Design review of the part built by this model. Coordinates are the model's own, in mm. Give positions to 0.01 mm unless a question says otherwise; leave off trailing zeros. Loops run counter-clockwise (first coordinate to the right, second up) from the corner with the lowest first, then second, coordinate; pieces in that order, holes last.
Autodesk Inventor part; units mm, degrees
ref_plane "YZ Plane" through (0, 0, 0) normal (1, 0, 0) x (0, 1, 0)
ref_plane "XZ Plane" through (0, 0, 0) normal (0, 1, 0) x (-1, 0, 0)
ref_plane "XY Plane" through (0, 0, 0) normal (0, 0, 1) x (1, 0, 0)
sketch "Sketch1" plane through (0, 0, 0) normal (0, 0, 1) x (1, 0, 0)
  line L0 (6, 225.5) -> (202, 225.5)
  line L1 (242, 185.5) -> (242, -10.5)
  line L2 (202, -50.5) -> (6, -50.5)
  line L3 (-34, -10.5) -> (-34, 185.5)
  line L4 (208, 237.5) -> (0, 237.5) construction
  line L5 (-46, 191.5) -> (-46, -16.5) construction
  arc A0 (0, 237.5) -> (-46, 191.5) centre (0, 191.5) ccw construction
  arc A1 (6, 225.5) -> (-34, 185.5) centre (6, 185.5) ccw
  arc A2 (242, 185.5) -> (202, 225.5) centre (202, 185.5) ccw
  arc A3 (202, -50.5) -> (242, -10.5) centre (202, -10.5) ccw
  arc A4 (-34, -10.5) -> (6, -50.5) centre (6, -10.5) ccw
  line L6 (51.5, 191.5) -> (16.5, 191.5)
  line L7 (16.5, 191.5) -> (16.5, 187.5)
  line L8 (51.5, 187.5) -> (16.5, 187.5)
  line L9 (51.5, 191.5) -> (51.5, 187.5)
  line L10 (121.5, 191.5) -> (86.5, 191.5)
  line L11 (86.5, 191.5) -> (86.5, 187.5)
  line L12 (121.5, 187.5) -> (86.5, 187.5)
  line L13 (121.5, 191.5) -> (121.5, 187.5)
  line L14 (191.5, 191.5) -> (156.5, 191.5)
  line L15 (156.5, 191.5) -> (156.5, 187.5)
  line L16 (191.5, 187.5) -> (156.5, 187.5)
  line L17 (191.5, 191.5) -> (191.5, 187.5)
  line L18 (208, 140) -> (208, 175)
  line L19 (208, 175) -> (204, 175)
  line L20 (204, 140) -> (204, 175)
  line L21 (208, 140) -> (204, 140)
  line L22 (208, 70) -> (208, 105)
  line L23 (208, 105) -> (204, 105)
  line L24 (204, 70) -> (204, 105)
  line L25 (208, 70) -> (204, 70)
  line L26 (208, 0) -> (208, 35)
  line L27 (208, 35) -> (204, 35)
  line L28 (204, 0) -> (204, 35)
  line L29 (208, 0) -> (204, 0)
  line L30 (156.5, -16.5) -> (191.5, -16.5)
  line L31 (191.5, -16.5) -> (191.5, -12.5)
  line L32 (156.5, -12.5) -> (191.5, -12.5)
  line L33 (156.5, -16.5) -> (156.5, -12.5)
  line L34 (86.5, -16.5) -> (121.5, -16.5)
  line L35 (121.5, -16.5) -> (121.5, -12.5)
  line L36 (86.5, -12.5) -> (121.5, -12.5)
  line L37 (86.5, -16.5) -> (86.5, -12.5)
  line L38 (16.5, -16.5) -> (51.5, -16.5)
  line L39 (51.5, -16.5) -> (51.5, -12.5)
  line L40 (16.5, -12.5) -> (51.5, -12.5)
  line L41 (16.5, -16.5) -> (16.5, -12.5)
  line L42 (0, 35) -> (0, 0)
  line L43 (0, 0) -> (4, 0)
  line L44 (4, 35) -> (4, 0)
  line L45 (0, 35) -> (4, 35)
  line L46 (0, 105) -> (0, 70)
  line L47 (0, 70) -> (4, 70)
  line L48 (4, 105) -> (4, 70)
  line L49 (0, 105) -> (4, 105)
  line L50 (0, 175) -> (0, 140)
  line L51 (0, 140) -> (4, 140)
  line L52 (4, 175) -> (4, 140)
  line L53 (0, 175) -> (4, 175)
  circle A5 centre (43, 152.5) radius 7.5
  line L54 (4, 180) -> (4, 165)
  line L55 (24, 7.5) -> (28, 7.5)
  line L56 (28, 7.5) -> (28, 47.5)
  line L57 (28, 47.5) -> (24, 47.5)
  line L58 (24, 47.5) -> (24, 7.5)
  line L59 (180, 7.5) -> (184, 7.5)
  line L60 (184, 7.5) -> (184, 47.5)
  line L61 (184, 47.5) -> (180, 47.5)
  line L62 (180, 47.5) -> (180, 7.5)
  line L63 (180, 127.5) -> (184, 127.5)
  line L64 (184, 127.5) -> (184, 167.5)
  line L65 (184, 167.5) -> (180, 167.5)
  line L66 (180, 167.5) -> (180, 127.5)
  line L67 (24, 127.5) -> (28, 127.5)
  line L68 (28, 127.5) -> (28, 167.5)
  line L69 (28, 167.5) -> (24, 167.5)
  line L70 (24, 167.5) -> (24, 127.5)
  line L71 (104, 187.5) -> (104, -12.5) construction
  circle A6 centre (26, 107.5) radius 1.5
  circle A7 centre (26, 67.5) radius 1.5
  circle A8 centre (182, 107.5) radius 1.5
  circle A9 centre (182, 67.5) radius 1.5
  line L72 (26, 127.5) -> (26, 107.5) construction
  line L73 (26, 67.5) -> (26, 47.5) construction
  line L74 (26, 107.5) -> (26, 87.5) construction
  line L75 (26, 87.5) -> (26, 67.5) construction
  line L76 (51.5, 191.5) -> (86.5, 187.5) construction
  line L77 (121.5, 187.5) -> (156.5, 191.5) construction
  circle A10 centre (69, 189.5) radius 1.5
  circle A11 centre (139, 189.5) radius 1.5
  circle A12 centre (2, 122.5) radius 1.5
  circle A13 centre (2, 52.5) radius 1.5
  circle A14 centre (69, -14.5) radius 1.5
  circle A15 centre (139, -14.5) radius 1.5
  circle A16 centre (206, 52.5) radius 1.5
  circle A17 centre (206, 122.5) radius 1.5
  point P0 (104, 237.5)
  point P1 (104, 225.5)
  point P2 (-34, 87.5)
  point P3 (-46, 87.5)
  point P4 (-24, 191.5)
  point P5 (4, 172.5)
  point P6 (182, 127.5)
  point P7 (182, 47.5)
  point P8 (104, 87.5)
  dimension "d0" = 10
  dimension "d2" = 40
  dimension "d4" = 15
  dimension "d6" = 4
  dimension "d7" = 40
  dimension "d9" = 20
  dimension "d10" = 4
  dimension "d11" = 40
  dimension "d12" = 4
  dimension "d13" = 40
  dimension "d14" = 4
  dimension "d15" = 40
  dimension "d16" = 20
  dimension "d17" = 15
  dimension "d18" = 15
  dimension "d19" = 20
  dimension "d22" = 3
  dimension "d24" = 3
  dimension "d27" = 360
extrude "Extrusion1" add sketch "Sketch1" along normal blind 4
properties part number "Cover" material "MDF Medium Density Fiberboard"
Q1. Take a section at C-C (z = 0.8). Give the number of separate pieces and of enclosed holes in the cut face, plus the area to 3 significant figures.
Results:
separate pieces: 1
enclosed holes: 29
area: 72,200 mm2
Q2. Insertion check: pin 1 (2 mm diameter, centred on x = 206, z = 2.5, fed in from -Y); pin 2 (1.2 mm diameter, centred on x = 207, z = 2, fed in from -Y); pin 3 (2 mm diameter, centred on y = 189, z = 3, fed in from +X). Each pin has a flat end and moves straight along its axis. Give the tip position at first contact, or say it passes through.
Results:
pin 1: stops at y = -50.39
pin 2: stops at y = -50.26
pin 3: stops at x = 241.92
Q3. Draft analysis for pull direction Y (two halves, no side actions). For faces 1 (the face through (230.594, -38.472, 1.972)), 2 (the face through (42.024, 145.064, 1.972)), 3 (the face through (102, 89, 4)), state which applies: pulls with the +Y half, pulls with the -Y half, needs draft (parallel to the pull), parting line crosses it, or undercut.
Results:
face 1: pulls with the -Y half
face 2: undercut
face 3: needs draft
Q4. Take a section at B-B (x = 43). Give the boundary of the cut face in (y, z).
Results:
outline: (-50.5, 0) - (-16.5, 0) - (-16.5, 4) - (-50.5, 4) - close; (-12.5, 0) - (145, 0) - (145, 4) - (-12.5, 4) - close; (160, 0) - (187.5, 0) - (187.5, 4) - (160, 4) - close; (191.5, 0) - (225.5, 0) - (225.5, 4) - (191.5, 4) - close
Q5. Wall thickness on line 1 (X direction, y = 32, z = 2.35); line 2 (Y direction, x = 120, z = 1.85); line 3 (X direction, y = 171, z = 1.2): over which ranges is each line inside the solid? List them lowest first.
Results:
line 1: x = -34 to 0, 4 to 24, 28 to 180, 184 to 204, 208 to 242
line 2: y = -50.5 to -16.5, -12.5 to 187.5, 191.5 to 225.5
line 3: x = -34 to 0, 4 to 204, 208 to 242
Q6. Take a section at A-A (y = 94). Give the boundary of the cut face in (x, z).
Results:
outline: (-34, 0) - (0, 0) - (0, 4) - (-34, 4) - close; (4, 0) - (204, 0) - (204, 4) - (4, 4) - close; (208, 0) - (242, 0) - (242, 4) - (208, 4) - close
Q7. Take a section at D-D (y = 206). Give the boundary of the cut face in (x, z).
Results:
outline: (-28.35, 0) - (236.35, 0) - (236.35, 4) - (-28.35, 4) - close
